Input: part model. Units: mm. Frame: model coordinates. Face numbers are marked on the shaded views. A direction names the side the tool comes from. Round coordinates to 2 decimals unless told otherwise and drop trailing zeros. Loops run counter-clockwise (first coordinate to the right, second up) from the corner with the lowest first, then second, coordinate; pieces in that order, holes last.
(1) Cut plane A-A, the plane z = 15. Output: boundary loops of the cut face in (x, y).
(2) Line query: line 1 (Z direction, x = 5, y = -0.5); line 2 (X direction, y = 1.25, z = 17.5); line 3 (Z direction, x = -1.75, y = -2). Output: solid intervals per line, ascending.
(3) Cut plane C-C, the plane z = -12.5. Output: boundary loops of the cut face in (x, y), and give its area (3 significant figures).
(4) Access query for the marked faces 4 and 5. Directions: +Z, -Z, +X, -X, +Y, -Y. A direction counts if a zero-diameter tool reaches every point of the face in a straight line with its end or side. Return the directions, or none.
(5) Cut plane B-B, the plane y = 0. Output: boundary loops of the cut face in (x, z), and give its area (3 significant figures).
(6) First-contact query: pin 1 Ø3 at (y, z) = (2, -11.5) entering from +X; pin 2 Ø4 at (x, z) = (3, -12.5) entering from -Y; pin 3 Ø2 at (x, y) = (0, -2) entering from +Z; pin 4 Ø6 at (x, y) = (2, -3) entering from -Z. Flat tips, straight axial feed; report the tip coordinate or a pass-through.
(7) Draft query along Y for the marked faces 1, 2 and 3. Return one class per face: released by +Y, released by -Y, zero draft, split by the parting line, or undercut.
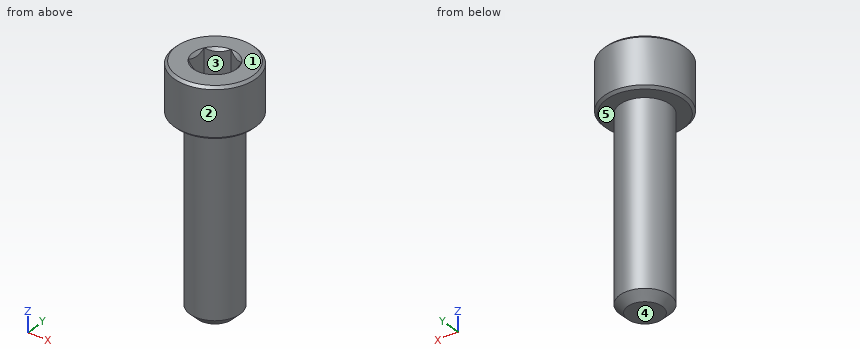
from build123d import *

# Parameters (mm, degrees)
CUT_EXTRUDE1_DEPTH = 7


with BuildPart() as part:
    # Sketch2 → Revolve1 (revolve)
    with BuildSketch(Plane(origin=(0, 0, 0), x_dir=(0, 0, -1), z_dir=(1, 0, 0))):
        Polygon((-19, 0), (-19, 6.1), (-18.6, 6.5), (-11.4, 6.5), (-11, 6.1), (-11, 4), (17.75, 4), (19, 2.75), (19, 0), align=None)
    revolve(axis=Axis((0, 0, -19), (0, 0, 1)))

    # Sketch3 → Cut-Extrude1 (cut)
    with BuildSketch(Plane.XY.offset(19)):
        Polygon((3, -1.732050808), (3, 1.732050808), (0, 3.464101615), (-3, 1.732050808), (-3, -1.732050808), (0, -3.464101615), align=None)
    extrude(amount=-CUT_EXTRUDE1_DEPTH, mode=Mode.SUBTRACT)

    # Cut-Extrude2 cone 1 section (through the dimple's axis) → Cut-Extrude2 (revolve, cut)
    with BuildSketch(Plane(origin=(0, 0, 19), x_dir=(0, -1, 0), z_dir=(1, 0, 0))):
        Polygon((0, 0), (3.464101615, 0), (0, 3.464101615), align=None)
    revolve(axis=Axis((0, 0, 19), (0, 0, -1)), mode=Mode.SUBTRACT)


solid = part.part
Reported:
1. outline: circle Ø13 at (0, 0); hole (-3, -1.73) - (0, -3.46) - (3, -1.73) - (3, 1.73) - (0, 3.46) - (-3, 1.73) - close
2. line 1: z = 11 to 19
2. line 2: x = -6.38 to -3, 3 to 6.38
2. line 3: z = -19 to 12
3. outline: circle Ø8 at (0, 0)
3. area: 50.3 mm2
4. face 4: -Z, +X, -X, +Y, -Y
4. face 5: -Z
5. outline: (-6.5, 11.4) - (-6.1, 11) - (-4, 11) - (-4, -17.75) - (-2.75, -19) - (2.75, -19) - (4, -17.75) - (4, 11) - (6.1, 11) - (6.5, 11.4) - (6.5, 18.6) - (6.1, 19) - (3.46, 19) - (3, 18.54) - (3, 12) - (-3, 12) - (-3, 18.54) - (-3.46, 19) - (-6.1, 19) - (-6.5, 18.6) - close
5. area: 300 mm2
6. pin 1: stops at x = 3.97
6. pin 2: stops at y = -3.87
6. pin 3: stops at z = 12
6. pin 4: stops at z = -19
7. face 1: zero draft
7. face 2: split by the parting line
7. face 3: undercut
